from build123d import *

# Parameters (mm, degrees)
SKETCH1_R           = 25
SKETCH1_R_2         = 23
EXTRUDE_THIN1_DEPTH = 30
SKETCH2_R           = 140
BOSS_EXTRUDE1_DEPTH = 2
SKETCH3_R           = 140
SKETCH3_R_2         = 138
BOSS_EXTRUDE2_DEPTH = 350
SKETCH4_R           = 140
BOSS_EXTRUDE3_DEPTH = 2


with BuildPart() as part:
    # Sketch1 → Extrude-Thin1 (new body)
    with BuildSketch(Plane(origin=(0, 0, 0), x_dir=(1, 0, 0), z_dir=(0, 1, 0))):
        Circle(SKETCH1_R)
        Circle(SKETCH1_R_2, mode=Mode.SUBTRACT)
    extrude(amount=EXTRUDE_THIN1_DEPTH)

    # Sketch2 → Boss-Extrude1 (add)
    with BuildSketch(Plane(origin=(0, 30, 0), x_dir=(1, 0, 0), z_dir=(0, 1, 0))):
        with Locations(Location((0, 0, 0), (0, 0, 270))):
            Circle(SKETCH2_R)
    extrude(amount=BOSS_EXTRUDE1_DEPTH)

    # Sketch3 → Boss-Extrude2 (add)
    with BuildSketch(Plane(origin=(0, 32, 0), x_dir=(1, 0, 0), z_dir=(0, 1, 0))):
        with Locations(Location((0, 0, 0), (0, 0, 270))):
            Circle(SKETCH3_R)
        with Locations(Location((0, 0, 0), (0, 0, 270))):
            Circle(SKETCH3_R_2, mode=Mode.SUBTRACT)
    extrude(amount=BOSS_EXTRUDE2_DEPTH)

    # Sketch4 → Boss-Extrude3 (add)
    with BuildSketch(Plane(origin=(0, 382, 0), x_dir=(1, 0, 0), z_dir=(0, 1, 0))):
        with Locations(Location((0, 0, 0), (0, 0, 270))):
            Circle(SKETCH4_R)
    extrude(amount=BOSS_EXTRUDE3_DEPTH)


solid = part.part
Model file for the job. Use its own axes, mm. A direction names the side the tool comes from. Give positions to 0.01 mm unless a question says otherwise; leave off trailing zeros. Order: outer loops, then holes, each group sorted by start corner. A loop starts at its lowest first (then second) coordinate and runs counter-clockwise, first axis right, second up. Notation, with made-up numbers: M 71,79 L 117,79 A20 cw 117,92 Z; hole C -28.5,-27 d9. An arc over 180 degrees is marked long. Write item = value, one per line.
Q1. Tool access for faces 1 (the flat face through (2, 32, -2)), 2 (the cylindrical face through (-2.994, 14.79, -22.804)), 3 (the flat face through (2, 384, -2)): list every direction of +Z, -Z, +X, -X, +Y, -Y with a clear straight run to the whole face (end or side of a thin tool).
Derived:
face_1 = none
face_2 = -Y
face_3 = +Z, -Z, +X, -X, +Y
Q2. Two-plate mould, pull along Z, no slides. Class faces 4 (the cylindrical face through (-85.19, 204.52, -111.1)), 5 (the cylindrical face through (6.068, 204.55, -137.867)), 6 (the flat face through (22.1, 0, 7.3)): pulls with the +Z half, pulls with the -Z half, needs draft (parallel to the pull), parting line crosses it, or undercut.
Derived:
face_4 = parting line crosses it
face_5 = undercut
face_6 = needs draft
Q3. Cut at D-D, the plane z = 123. List the corners of the cut face in (x, y).
Derived:
outline = M -66.87,30 L 66.87,30 L 66.87,384 L -66.87,384 Z; hole M -62.57,32 L 62.57,32 L 62.57,382 L -62.57,382 Z
Q4. Cut at C-C, the plane y = 110.5. List the corners of the cut face in (x, z).
Derived:
outline = C 0,0 d280; hole C 0,0 d276
Q5. Flat gauge pins, fed straight in: pin 1 (2 mm diameter, centred on x = -21.5, y = 150.5, fed in from -Z); pin 2 (2 mm diameter, centred on y = 78.5, z = -17.5, fed in from -X); pin 3 (3 mm diameter, centred on x = -101, y = 334.5, fed in from +Z). Where does each tip first touch, or does it go through?
Derived:
pin_1 = -138.49
pin_2 = -139.02
pin_3 = 98.49
Q6. Cut at A-A, the plane z = 0. List the corners of the cut face in (x, y), then the cut area to 3 significant figures.
Derived:
outline = M -140,30 L -25,30 L -25,0 L -23,0 L -23,30 L 23,30 L 23,0 L 25,0 L 25,30 L 140,30 L 140,384 L -140,384 Z; hole M -138,32 L 138,32 L 138,382 L -138,382 Z
area = 2,640 mm2
Q7. Drill centre lines: line 1 (Y direction, x = -77, z = 46.5); line 2 (X direction, y = 10.5, z = 0). Where is each one in solid material? Low to high. Write a range as [from, to].
Derived:
line_1 = [30, 32], [382, 384]
line_2 = [-25, -23], [23, 25]
Q8. Cut at B-B, the plane x = 0. List the corners of the cut face in (y, z), then the cut area to 3 significant figures.
Derived:
outline = M 0,-25 L 30,-25 L 30,-140 L 384,-140 L 384,140 L 30,140 L 30,25 L 0,25 L 0,23 L 30,23 L 30,-23 L 0,-23 Z; hole M 32,-138 L 382,-138 L 382,138 L 32,138 Z
area = 2,640 mm2
